Study the drawing (mm; zero at the part's minimum x, y, z) and answer. A direction names the side the tool comes from. Give positions to 0.01 mm unless a question says otherwise; leave off trailing zeros. Write each loop counter-clockwise with the first axis right and the second up, starting at its lowest first coordinate (ties: lowest second). Pieces come first, ordered by that corner, then holes. Notation, with made-up numbers: M -14.5,78 L 37.5,78 A34 ccw 37.5,114 Z; hole C 70,-14 d10. An arc over 180 degrees is marked long. Use a Markdown table: item, result. Add a question column.
Item 1: A cutting plane is placed at B-B on z = 5.5. Determine the outline of the cut face in (x, y), then the cut area to 3 significant figures.
Item 2: Consider probe 1 along Y at (x, z) = (13.75, 3.5); probe 2 along Y at (x, z) = (4, 9.25); probe 3 along Z at (x, y) = (8, 26). Determine where each line is inside the solid, lowest interval first. Write a range as [from, to].
Item 3: A cutting plane is placed at C-C on y = 13. Determine the outline of the cut face in (x, z).
Item 4: For the marked faces 1, 2, 3 and 4, determine the directions among +Z, -Z, +X, -X, +Y, -Y from which every point of the face is accessible in a straight line to the end or side of a thin tool.
Item 5: Given P1, Ø1, axis at x = 5.5, z = 3, coming from the +Y side; P2, Ø3, axis at x = 5, y = 11, coming from the +Z side; P3, Ø2, axis at y = 22, z = 9.5, coming from the -X side, each flat-ended and moving along its own axis, determine where each tip first touches the part or whether it passes through.
Item 6: A cutting plane is placed at A-A on x = 9.5. Determine the outline of the cut face in (y, z).
Item 7: A cutting plane is placed at D-D on z = 11.5. Determine the outline of the cut face in (x, y).
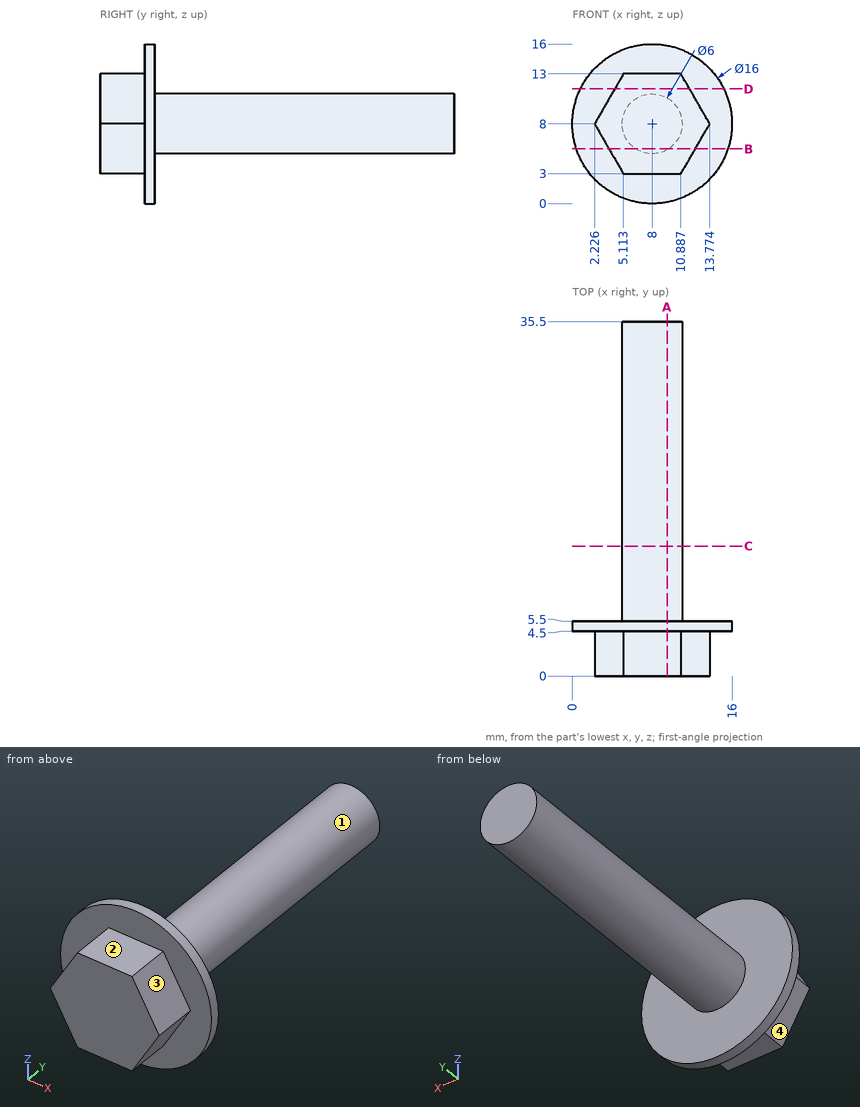
Filled in:
| question | item | result |
|---|---|---|
| 1 | outline | M 0.4,4.5 L 3.67,4.5 L 3.67,0 L 12.33,0 L 12.33,4.5 L 15.6,4.5 L 15.6,5.5 L 9.66,5.5 L 9.66,35.5 L 6.34,35.5 L 6.34,5.5 L 0.4,5.5 Z |
| 1 | area | 154 mm² |
| 2 | probe 1 | [4.5, 5.5] |
| 2 | probe 2 | [0, 5.5] |
| 2 | probe 3 | [5, 11] |
| 3 | outline | C 8,8 d6 |
| 4 | face 1 | +Y |
| 4 | face 2 | +Z, +X, -X, -Y |
| 4 | face 3 | +Z, +X, -Y |
| 4 | face 4 | -Z, -X, -Y |
| 5 | P1 | y = 5.5 |
| 5 | P2 | z = 10.6 |
| 5 | P3 | x = 5.04 |
| 6 | outline | M 0,3 L 4.5,3 L 4.5,0.14 L 5.5,0.14 L 5.5,5.4 L 35.5,5.4 L 35.5,10.6 L 5.5,10.6 L 5.5,15.86 L 4.5,15.86 L 4.5,13 L 0,13 Z |
| 7 | outline | M 0.81,4.5 L 4.25,4.5 L 4.25,0 L 11.75,0 L 11.75,4.5 L 15.19,4.5 L 15.19,5.5 L 0.81,5.5 Z |
